Build history of the part. All positions in model axes, mm. Give positions to 0.01 mm unless a question says otherwise; leave off trailing zeros. Write each loop counter-clockwise with the first axis right and the second up, starting at its lowest first coordinate (ties: lowest second). Pieces come first, ordered by that corner, then holes. Notation, with made-up numbers: (85, -1) -> (137, -1) arc R16 ccw to (137, 30) -> close; hole circle Ø10 at (4, -18). An arc over 180 degrees is marked (long way). Put each result on its own line as item: value. Start each with the question number.
Item 1: Flat gauge pins, fed straight in: pin 1 Ø4 at (y, z) = (5, -0.5) entering from +X; pin 2 Ø5 at (y, z) = (5, 63) entering from -X; pin 3 Ø3 at (x, y) = (51.5, 5) entering from +Z; pin 4 Ø5.5 at (x, z) = (-12.5, 49.34) entering from -Y. Where does each tip first touch, or does it go through?
Item 2: Slice it at A-A, the plane x = 12.5. List the corners of the cut face in (y, z), plus the area to 3 significant figures.
Item 3: Slice it at B-B, the plane y = 1.75. Give the number of separate pieces and of enclosed holes in the cut face, plus the area to 3 significant figures.
Item 4: Slice it at D-D, the plane z = -61.5. List the corners of the cut face in (x, y).
Item 5: Drill centre lines: line 1 along Z through (x, y) = (-12.5, 2.75); line 2 along Z through (x, y) = (-12.5, 8.8); line 3 along X through (y, z) = (6.25, 47). Where is each one in solid material? Low to high.
Item 6: Slice it at C-C, the plane z = 62.5. List the corners of the cut face in (x, y).
Autodesk Inventor part; units mm, degrees
ref_plane "YZ Plane" through (0, 0, 0) normal (1, 0, 0) x (0, 1, 0)
ref_plane "XZ Plane" through (0, 0, 0) normal (0, 1, 0) x (-1, 0, 0)
ref_plane "XY Plane" through (0, 0, 0) normal (0, 0, 1) x (1, 0, 0)
sketch "Sketch1" plane through (0, 0, 0) normal (0, 1, 0) x (-1, 0, 0)
  arc A0 (-44.5, -7) -> (-44.5, 7) centre (-44.5, 0) ccw
  arc A1 (44.5, 7) -> (44.5, -7) centre (44.5, 0) ccw
  line L0 (44.5, 7) -> (59.6236, 7)
  line L1 (44.5, -7) -> (60, -7)
  line L2 (-44.5, 7) -> (-60, 7)
  line L3 (-44.5, -7) -> (-60, -7)
  line L4 (60, -7) -> (60, -19.5)
  line L5 (-60, 7) -> (-60, 19.5)
  line L6 (59.6236, 7) -> (59.6236, 19.5)
  line L7 (-60, -7) -> (-60, -19.5)
  line L8 (37.5, -90.6623) -> (-37.5, -90.6623)
  line L9 (17.5, 94.3377) -> (-17.5, 94.3377)
  line L10 (60, -19.5) -> (37.5, -42)
  line L11 (-60, -19.5) -> (-37.5, -42)
  line L12 (37.5, -90.6623) -> (37.5, -42)
  line L13 (-37.5, -90.6623) -> (-37.5, -42)
  line L14 (59.6236, 19.5) -> (37.5, 41.6236)
  line L15 (-60, 19.5) -> (-37.8764, 41.6236)
  line L16 (37.5, 41.6236) -> (37.5, 74.3377)
  line L17 (-37.8764, 41.6236) -> (-37.8764, 73.9613)
  line L18 (17.5, 94.3377) -> (37.5, 74.3377)
  line L19 (-17.5, 94.3377) -> (-37.8764, 73.9613)
  point P0 (0, 0)
  dimension "d0" = 89
  dimension "d1" = 44.5
  dimension "d5" = 60
  dimension "d10" = 39
  dimension "d11" = 19.5
  dimension "d12" = 19.5
  dimension "d13" = 39
  dimension "d14" = 19.5
  dimension "d15" = 19.5
  dimension "d16" = 75
  dimension "d17" = 37.5
  dimension "d18" = 35
  dimension "d19" = 17.5
  dimension "d20" = 185
  dimension "d22" = 45
  dimension "d23" = 45
  dimension "d24" = 45
  dimension "d25" = 45
  dimension "d28" = 45
  dimension "d29" = 45
extrude "Extrusion1" add sketch "Sketch1" along normal blind 10
sketch "Sketch2" plane through (0, 10, 0) normal (0, 1, 0) x (1, 0, 0)
  circle A0 centre (-12.5, 40.6623) radius 5.5
  circle A1 centre (-12.5, -4.3377) radius 5.5
  circle A2 centre (-12.5, -49.3377) radius 5.5
  line L0 (37.5, 90.6623) -> (-37.5, 90.6623)
  circle A3 centre (12.5, -49.3377) radius 5.5
  circle A4 centre (12.5, -4.3377) radius 5.5
  circle A5 centre (12.5, 40.6623) radius 5.5
  point P0 (0, 0)
  dimension "d32" = 11
  dimension "d33" = 11
  dimension "d34" = 11
  dimension "d35" = 50
  dimension "d36" = 45
  dimension "d37" = 45
  dimension "d38" = 11
  dimension "d39" = 11
  dimension "d40" = 11
  dimension "d41" = 25
  dimension "d42" = 12.5
  dimension "d43" = 12.5
  dimension "d44" = 12.5
  dimension "d45" = 12.5
  dimension "d46" = 12.5
extrude "Extrusion2" cut sketch "Sketch2" against normal blind 6
sketch "Sketch3" plane through (-12.5, 4, 4.3377) normal (0, 1, 0) x (1, 0, 0)
  circle A0 centre (0, 0) radius 3
  circle A1 centre (25, 0) radius 5.5
  circle A2 centre (25, 0) radius 3
  circle A3 centre (0, -45) radius 5.5
  circle A4 centre (0, -45) radius 3
  circle A5 centre (0, 45) radius 5.5
  circle A6 centre (25, 45) radius 5.5
  circle A7 centre (25, -45) radius 3
  circle A8 centre (25, 45) radius 3
  circle A9 centre (0, 45) radius 3
  point P0 (12.5, 4.3377)
  dimension "d51" = 6
  dimension "d52" = 6
  dimension "d53" = 6
  dimension "d55" = 6
  dimension "d56" = 6
  dimension "d57" = 6
extrude "Extrusion3" cut sketch "Sketch3" against normal blind 6 contours A0 | A2 | A4 | A7 | A8 | A9
fillet "Fillet1" radius 2 1 edges at (-37.5, 5, -90.6623)
fillet "Fillet2" radius 2 1 edges at (37.5, 5, -90.6623)
properties part number "Groundplate"
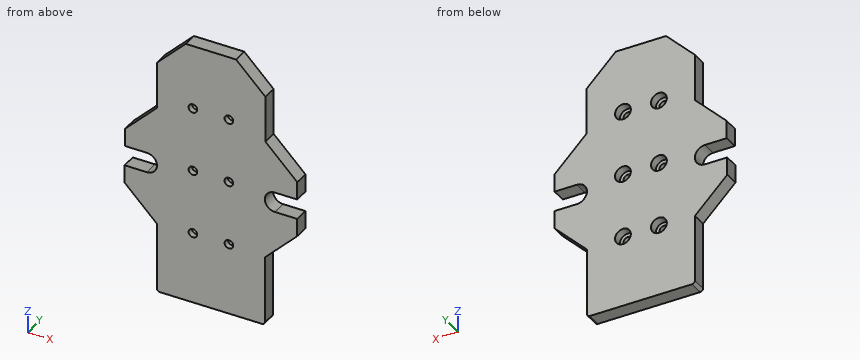
Values follow:
1. pin 1: x = 37.96
1. pin 2: x = -37.5
1. pin 3: z = 29.5
1. pin 4: through
2. outline: (0, -90.66) -> (10, -90.66) -> (10, -46.16) -> (4, -46.16) -> (4, -43.66) -> (0, -43.66) -> close; (0, -37.66) -> (4, -37.66) -> (4, -35.16) -> (10, -35.16) -> (10, -1.16) -> (4, -1.16) -> (4, 1.34) -> (0, 1.34) -> close; (0, 7.34) -> (4, 7.34) -> (4, 9.84) -> (10, 9.84) -> (10, 43.84) -> (4, 43.84) -> (4, 46.34) -> (0, 46.34) -> close; (0, 52.34) -> (4, 52.34) -> (4, 54.84) -> (10, 54.84) -> (10, 94.34) -> (0, 94.34) -> close
2. area: 1,580 mm2
3. separate pieces: 1
3. enclosed holes: 6
3. area: 15,500 mm2
4. outline: (-37.5, 0) -> (37.5, 0) -> (37.5, 10) -> (-37.5, 10) -> close
5. line 1: -90.66 to -43.66, -37.66 to 1.34, 7.34 to 46.34, 52.34 to 94.34
5. line 2: -90.66 to -46.16, -35.16 to -1.16, 9.84 to 43.84, 54.84 to 94.34
5. line 3: -37.5 to -17.48, -7.52 to 7.52, 17.48 to 37.88
6. outline: (-37.5, 0) -> (37.88, 0) -> (37.88, 10) -> (-37.5, 10) -> close
